Check sheet for the modelled part. Datum: model origin and axes. Units: mm. A direction names the side the tool comes from. Give positions to 0.01 mm unless a question says otherwise; leave off trailing zeros. Loops run counter-clockwise (first coordinate to the right, second up) from the corner with the lowest first, then second, coordinate; pieces in that order, holes last. Notation, with made-up numbers: (20, -31.75) -> (62, -31.75) arc R30 ccw to (62, -7.75) -> close; hole circle Ø7 at (39, -20.5). An arc over 180 degrees is marked (long way). Write each question's results on one line, items separated by ' | '. Start each with the question number.
Item 1: Cross-section at A-A on y = 10. Enter the section's corners in (x, z), then the cut area to 3 significant figures.
Item 2: Gauge pin test, flat ends, axial feed: pin 1 Ø0.9 at (y, z) = (22, -5) entering from -X; pin 2 Ø2 at (x, z) = (-4.5, -4) entering from -Y; pin 3 Ø0.8 at (x, z) = (-1, -10.5) entering from -Y; pin 4 Ø3 at (y, z) = (10, -7.5) entering from -X. Record the tip position at first contact, or that the pin passes through.
Item 3: Cross-section at C-C on z = -7.5. Enter the section's corners in (x, y).
Item 4: Cross-section at D-D on z = -10.75. Enter the section's corners in (x, y).
Item 5: Cross-section at B-B on x = -2. Enter the section's corners in (y, z).
Item 6: Scan lines: line 1 along Y through (x, z) = (-1.25, -5.25); line 2 along Y through (x, z) = (1.4, -7.5); line 3 along X through (y, z) = (23, -1). Record each from-to range of solid material in increasing order.
Item 7: Access from +Z, -Z, +X, -X, +Y, -Y to the whole of each face (thin tool, end or side, straight path). Record for faces 1 (the face through (-1.5, 22, -8)), 2 (the face through (-3, 27, -5)), 3 (the face through (-1, 23.5, -2)), 4 (the face through (-1, 40, -9)), 5 (the face through (-3, 28.25, -4)).
Item 8: Mould release check, pull along Y, two halves, no side actions. Record for faces 6 (the face through (3, 20, -7)), 7 (the face through (1, 0, -7)), 8 (the face through (-3, 35.25, -4)): pulls with the +Y half, pulls with the -Y half, needs draft (parallel to the pull), parting line crosses it, or undercut.
from build123d import *

# Parameters (mm, degrees)
SKETCH1_W           = 15
SKETCH1_H           = 40
SKETCH1_R           = 2.6
BOSS_EXTRUDE1_DEPTH = 3
SKETCH2_W           = 15
SKETCH2_H           = 3
BOSS_EXTRUDE2_DEPTH = 1.5
BOSS_EXTRUDE3_DEPTH = 6
SKETCH4_W           = 2
SKETCH4_H           = 7
CUT_EXTRUDE1_DEPTH  = 6


with BuildPart() as part:
    # Sketch1 → Boss-Extrude1 (new body)
    with BuildSketch(Plane(origin=(0, 0, 0), x_dir=(0, 0, -1), z_dir=(1, 0, 0))):
        with Locations((7.5, 20)):
            Rectangle(SKETCH1_W, SKETCH1_H)
        with Locations((7.5, 10)):
            Circle(SKETCH1_R, mode=Mode.SUBTRACT)
    extrude(amount=BOSS_EXTRUDE1_DEPTH)

    # Sketch2 → Boss-Extrude2 (add)
    with BuildSketch(Plane.ZY):
        with Locations((-7.5, 22)):
            Rectangle(SKETCH2_W, SKETCH2_H)
    extrude(amount=BOSS_EXTRUDE2_DEPTH)

    # Sketch3 → Boss-Extrude3 (add)
    with BuildSketch(Plane.ZY):
        Polygon((-15, 25), (-5, 25), (-5, 38.5), (-15, 38.5), (-15, 40), (-3, 40), (-3, 23.5), (-15, 23.5), align=None)
    extrude(amount=BOSS_EXTRUDE3_DEPTH)

    # Sketch4 → Cut-Extrude1 (cut)
    with BuildSketch(Plane.ZY.offset(6)):
        with Locations((-4, 31.75)):
            Rectangle(SKETCH4_W, SKETCH4_H)
    extrude(amount=-CUT_EXTRUDE1_DEPTH, mode=Mode.SUBTRACT)


solid = part.part
Answer sheet:
1) outline: (0, -15) -> (3, -15) -> (3, -10.1) -> (0, -10.1) -> close; (0, -4.9) -> (3, -4.9) -> (3, 0) -> (0, 0) -> close | area: 29.4 mm²
2) pin 1: stops at x = -1.5 | pin 2: stops at y = 23.5 | pin 3: stops at y = 20.5 | pin 4: passes through
3) outline: (-6, 23.5) -> (-1.5, 23.5) -> (-1.5, 20.5) -> (0, 20.5) -> (0, 12.6) -> (3, 12.6) -> (3, 40) -> (-6, 40) -> (-6, 38.5) -> (0, 38.5) -> (0, 25) -> (-6, 25) -> close; (0, 0) -> (3, 0) -> (3, 7.4) -> (0, 7.4) -> close
4) outline: (-6, 23.5) -> (-1.5, 23.5) -> (-1.5, 20.5) -> (0, 20.5) -> (0, 0) -> (3, 0) -> (3, 40) -> (-6, 40) -> (-6, 38.5) -> (0, 38.5) -> (0, 25) -> (-6, 25) -> close
5) outline: (23.5, -15) -> (25, -15) -> (25, -5) -> (28.25, -5) -> (28.25, -3) -> (23.5, -3) -> close; (35.25, -5) -> (38.5, -5) -> (38.5, -15) -> (40, -15) -> (40, -3) -> (35.25, -3) -> close
6) line 1: y = 20.5 to 25, 38.5 to 40 | line 2: y = 0 to 7.4, 12.6 to 40 | line 3: x = -1.5 to 3
7) face 1: +Z, -Z, -X, -Y | face 2: -Z, -X | face 3: +Z, -X, +Y | face 4: +Z, -Z, +X, -X, +Y | face 5: +Z, -Z, -X
8) face 6: needs draft | face 7: pulls with the -Y half | face 8: undercut
